The listing builds one solid part. Answer for the finished solid, in the listing's coordinates (mm). A direction names the side the tool comes from. Coordinates: 2 decimals unless noted, no trailing zeros. Order: outer loops, then holes, each group sorted by start corner. A loop starts at its lowest first (then second) coordinate and runs counter-clockwise, first axis right, second up. Notation, with made-up numbers: (-39.75, 85.5) -> (18.25, 85.5) arc R19 ccw to (18.25, 90.5) -> close; hole circle Ø11 at (-30.75, 33). An arc over 180 degrees is marked (long way). Return JSON: item names as keys, results as strings.
```python
from build123d import *

# Parameters (mm, degrees)
SKETCH2_R           = 2.6
SKETCH2_R_2         = 12.75
BOSS_EXTRUDE1_DEPTH = 5
SKETCH3_W           = 115
SKETCH3_H           = 100
BOSS_EXTRUDE2_DEPTH = 5
SKETCH4_W           = 165
SKETCH4_H           = 28.75
BOSS_EXTRUDE3_DEPTH = 5
SKETCH5_W           = 3
SKETCH5_H           = 95
SKETCH5_H_2         = 25
BOSS_EXTRUDE4_DEPTH = 23.75
SKETCH6_R           = 4
CUT_EXTRUDE1_DEPTH  = 5
SKETCH7_R           = 2.55
CUT_EXTRUDE2_DEPTH  = 1
SKETCH8_R           = 2.15
CUT_EXTRUDE3_DEPTH  = 4
SKETCH9_W           = 3
SKETCH9_H           = 28.75
BOSS_EXTRUDE5_DEPTH = 100
CHAMFER1_SIZE       = 70
CHAMFER1_SIZE2      = 28.709092262
FILLET1_R           = 5
FILLET2_R           = 2.5
CUT_EXTRUDE4_DEPTH  = 1.25


with BuildPart() as part:
    # Sketch2 → Boss-Extrude1 (new body)
    with BuildSketch(Plane.XZ.offset(-21.878326304)):
        Polygon((119.866549827, 74.413081659), (14.866549827, 74.413081659), (4.866549827, 74.413081659), (4.866549827, 21.913081659), (14.866549827, 21.913081659), (119.866549827, 21.913081659), align=None)
        Polygon((9.316549827, 34.313081659), (14.316549827, 34.313081659), (26.316549827, 34.313081659), (57.316549827, 34.313081659), (64.316549827, 34.313081659), (64.316549827, 31.013081659), (57.316549753, 31.013081659), (26.316549827, 31.013081659), (14.316549827, 31.013081659), (9.316549827, 31.013081659), align=None, mode=Mode.SUBTRACT)
        with Locations((76.704406531, 39.438081659)):
            Circle(SKETCH2_R, mode=Mode.SUBTRACT)
        with Locations((106.928693123, 39.438081659)):
            Circle(SKETCH2_R, mode=Mode.SUBTRACT)
        Polygon((13.816549827, 59.663081659), (16.816549827, 59.663081659), (59.816549827, 59.663081659), (59.816549827, 36.663081659), (16.816549827, 36.663081659), (13.816549827, 36.663081659), align=None, mode=Mode.SUBTRACT)
        Polygon((57.316549827, 65.313081659), (64.316549827, 65.313081659), (64.316549827, 62.013081659), (57.316549827, 62.013081659), (26.316549827, 62.013081659), (14.316549827, 62.013081659), (9.316549827, 62.013081659), (9.316549827, 65.313081659), (14.316549827, 65.313081659), (26.316549827, 65.313081659), align=None, mode=Mode.SUBTRACT)
        with Locations((91.816549827, 48.163081659)):
            Circle(SKETCH2_R_2, mode=Mode.SUBTRACT)
        with Locations((91.816549827, 65.613081659)):
            Circle(SKETCH2_R, mode=Mode.SUBTRACT)
    extrude(amount=BOSS_EXTRUDE1_DEPTH)

    # Sketch3 → Boss-Extrude2 (add)
    with BuildSketch(Plane(origin=(0, 0, 21.913081659), x_dir=(-1, 0, 0), z_dir=(0, 0, -1))):
        with Locations((-62.366549827, 66.878326304)):
            Rectangle(SKETCH3_W, SKETCH3_H)
    extrude(amount=BOSS_EXTRUDE2_DEPTH)

    # Sketch4 → Boss-Extrude3 (add)
    with BuildSketch(Plane(origin=(0, 116.878326304, 0), x_dir=(1, 0, 0), z_dir=(0, 1, 0))):
        with Locations((62.366549827, -31.288081659)):
            Rectangle(SKETCH4_W, SKETCH4_H)
    extrude(amount=BOSS_EXTRUDE3_DEPTH)

    # Sketch5 → Boss-Extrude4 (add)
    with BuildSketch(Plane.XY.offset(21.913081659)):
        with Locations((65.816549827, 69.378326304)):
            Rectangle(SKETCH5_W, SKETCH5_H)
        with Locations((118.366549827, 104.378326304)):
            Rectangle(SKETCH5_W, SKETCH5_H_2)
        with Locations((118.366549827, 34.378326304)):
            Rectangle(SKETCH5_W, SKETCH5_H_2)
        with Locations((6.366549827, 34.378326304)):
            Rectangle(SKETCH5_W, SKETCH5_H_2)
        with Locations((6.366549827, 104.378326304)):
            Rectangle(SKETCH5_W, SKETCH5_H_2)
    extrude(amount=BOSS_EXTRUDE4_DEPTH)

    # Sketch6 → Cut-Extrude1 (cut)
    with BuildSketch(Plane(origin=(0, 121.878326304, 0), x_dir=(1, 0, 0), z_dir=(0, 1, 0))):
        with Locations((134.866549827, -31.288081659)):
            Circle(SKETCH6_R)
        with Locations((-10.133450173, -31.288081659)):
            Circle(SKETCH6_R)
    extrude(amount=-CUT_EXTRUDE1_DEPTH, mode=Mode.SUBTRACT)

    # Sketch7 → Cut-Extrude2 (cut)
    with BuildSketch(Plane(origin=(0, 0, 16.913081659), x_dir=(-1, 0, 0), z_dir=(0, 0, -1))):
        with Locations((-105.165549827, 90.587326304)):
            Circle(SKETCH7_R)
        with Locations((-105.165549827, 48.423326304)):
            Circle(SKETCH7_R)
        with Locations((-19.821549827, 48.423326304)):
            Circle(SKETCH7_R)
        with Locations((-19.821549827, 90.587326304)):
            Circle(SKETCH7_R)
    extrude(amount=-CUT_EXTRUDE2_DEPTH, mode=Mode.SUBTRACT)

    # Sketch8 → Cut-Extrude3 (cut)
    with BuildSketch(Plane(origin=(0, 0, 17.913081659), x_dir=(-1, 0, 0), z_dir=(0, 0, -1))):
        with Locations((-105.165549827, 90.587326304)):
            Circle(SKETCH8_R)
        with Locations((-19.825549827, 90.587326304)):
            Circle(SKETCH8_R)
        with Locations((-19.825549827, 48.427326304)):
            Circle(SKETCH8_R)
        with Locations((-105.165549827, 48.427326304)):
            Circle(SKETCH8_R)
    extrude(amount=-CUT_EXTRUDE3_DEPTH, mode=Mode.SUBTRACT)

    # Sketch9 → Boss-Extrude5 (add)
    with BuildSketch(Plane(origin=(0, 21.878326304, 0), x_dir=(1, 0, 0), z_dir=(0, 1, 0))):
        with Locations((65.816549827, -60.038081659)):
            Rectangle(SKETCH9_W, SKETCH9_H)
    extrude(amount=BOSS_EXTRUDE5_DEPTH)

    # Chamfer1
    chamfer1_edges = [part.edges().sort_by_distance(p)[0] for p in [
        (65.816549827, 121.878326304, 74.413081659),
    ]]
    chamfer1_side = [part.faces().sort_by_distance(p)[0] for p in [
        (118.309308677, 19.378326304, 74.413081659),
    ]]
    chamfer(chamfer1_edges, length=CHAMFER1_SIZE, length2=CHAMFER1_SIZE2, reference=chamfer1_side[0])

    # Fillet1
    fillet1_edges = [part.edges().sort_by_distance(p)[0] for p in [
        (67.316549827, 116.878326304, 33.788081659),
        (64.316549827, 116.878326304, 33.788081659),
        (118.366549827, 91.878326304, 45.663081659),
        (118.366549827, 91.878326304, 21.913081659),
        (116.866549827, 116.878326304, 33.788081659),
        (118.366549827, 46.878326304, 45.663081659),
        (118.366549827, 46.878326304, 21.913081659),
        (6.366549827, 46.878326304, 45.663081659),
        (6.366549827, 46.878326304, 21.913081659),
        (7.866549827, 116.878326304, 33.788081659),
        (6.366549827, 91.878326304, 45.663081659),
        (6.366549827, 91.878326304, 21.913081659),
        (119.866549827, 19.378326304, 74.413081659),
        (4.866549827, 19.378326304, 74.413081659),
        (119.866549827, 116.878326304, 31.288081659),
        (4.866549827, 116.878326304, 31.288081659),
        (-20.133450173, 119.378326304, 16.913081659),
        (-20.133450173, 119.378326304, 45.663081659),
        (144.866549827, 119.378326304, 45.663081659),
        (144.866549827, 119.378326304, 16.913081659),
    ]]
    fillet(fillet1_edges, radius=FILLET1_R)

    # Fillet2
    fillet2_edges = [part.edges().sort_by_distance(p)[0] for p in [
        (118.366549827, 21.878326304, 45.663081659),
        (6.366549827, 21.878326304, 45.663081659),
        (119.866549827, 16.878326304, 43.163081659),
        (4.866549827, 16.878326304, 43.163081659),
        (62.366549827, 16.878326304, 74.413081659),
        (118.402083733, 16.878326304, 72.948615565),
        (6.331015921, 16.878326304, 72.948615565),
        (62.366549827, 16.878326304, 16.913081659),
    ]]
    fillet(fillet2_edges, radius=FILLET2_R)

    # Sketch10 → Cut-Extrude4 (cut)
    with BuildSketch(Plane(origin=(0, 21.878326304, 0), x_dir=(1, 0, 0), z_dir=(0, 1, 0))):
        Polygon((106.849185334, -35.980469853), (103.894559568, -37.778131521), (103.974067356, -41.235743327), (107.008200912, -42.895693466), (109.962826678, -41.098031798), (109.883318889, -37.640419991), align=None)
        Polygon((73.749780764, -41.235743327), (76.78391432, -42.895693466), (79.738540086, -41.098031798), (79.659032297, -37.640419991), (76.624898742, -35.980469853), (73.670272976, -37.778131521), align=None)
        Polygon((94.850683382, -67.273031798), (94.771175593, -63.815419991), (91.737042038, -62.155469853), (88.782416272, -63.953131521), (88.86192406, -67.410743327), (91.896057616, -69.070693466), align=None)
    extrude(amount=-CUT_EXTRUDE4_DEPTH, mode=Mode.SUBTRACT)


solid = part.part
```
Item 1: Flat-ended cylindrical pins translate along their axes: pin 1 (4 mm diameter, centred on x = 76.7, z = 39.44, fed in from -Y); pin 2 (4.5 mm diameter, centred on x = 19.82, y = 48.42, fed in from +Z); pin 3 (12 mm diameter, centred on x = 41.5, z = 66, fed in from +Y). Find the tip coordinate at first contact, or state that the pin passes through.
Answer list:
{"pin 1": "y = 116.88", "pin 2": "z = 21.91", "pin 3": "y = 21.88"}
Item 2: The part is cut by section D-D on x = 126.5. Determine the outline of the cut face in (y, z), plus the area to 3 significant figures.
Answer list:
{"outline": "(116.88, 16.91) -> (121.88, 16.91) -> (121.88, 45.66) -> (116.88, 45.66) -> close", "area": "144 mm2"}
Item 3: The part is cut by section C-C on y = 108.5. Determine the outline of the cut face in (x, z), plus the area to 3 significant figures.
Answer list:
{"outline": "(4.87, 16.91) -> (119.87, 16.91) -> (119.87, 45.66) -> (116.87, 45.66) -> (116.87, 21.91) -> (67.32, 21.91) -> (67.32, 51.19) -> (64.32, 51.19) -> (64.32, 21.91) -> (7.87, 21.91) -> (7.87, 45.66) -> (4.87, 45.66) -> close", "area": "805 mm2"}
Item 4: Find the intervals of material crossed by probe 1 along X at (y, z) = (44.5, 32.5); probe 2 along Y at (x, z) = (45, 24.5); probe 3 along X at (y, z) = (68, 43), in increasing order.
Answer list:
{"probe 1": "4.87 to 7.87, 64.32 to 67.32, 116.87 to 119.87", "probe 2": "16.88 to 21.88, 116.88 to 121.88", "probe 3": "64.32 to 67.32"}
Item 5: The part is cut by section A-A on x = 40. Determine the outline of the cut face in (y, z).
Answer list:
{"outline": "(16.88, 19.41) arc R2.5 ccw to (19.38, 16.91) -> (121.88, 16.91) -> (121.88, 45.66) -> (116.88, 45.66) -> (116.88, 21.91) -> (21.88, 21.91) -> (21.88, 31.01) -> (16.88, 31.01) -> close; (16.88, 34.31) -> (21.88, 34.31) -> (21.88, 36.66) -> (16.88, 36.66) -> close; (16.88, 59.66) -> (21.88, 59.66) -> (21.88, 62.01) -> (16.88, 62.01) -> close; (16.88, 65.31) -> (21.88, 65.31) -> (21.88, 74.41) -> (19.38, 74.41) arc R2.5 ccw to (16.88, 71.91) -> close"}
Item 6: Which of the six approach directions +Z, -Z, +X, -X, +Y, -Y give full straight-line access (tool end or side, diameter ignored) to faces 1 (the cylindrical face through (6.39, 48.38, 23.34)), 2 (the flat face through (4.867, 62, 20)), 3 (the flat face through (74, 20.628, 38)), 4 (the flat face through (7.867, 102, 34))?
Answer list:
{"face 1": "+Z, -X", "face 2": "+Z, -Z, -X, -Y", "face 3": "none", "face 4": "+Z"}
Item 7: Determine the mould class of faces 5 (the cylindrical face through (3.441, 115.375, 31.087)), 6 (the cylindrical face through (20.29, 46.33, 19.89)), 7 (the flat face through (106, 118, 45.663)) for opening direction Y: pulls with the +Y half, pulls with the -Y half, needs draft (parallel to the pull), parting line crosses it, or undercut.
Answer list:
{"face 5": "pulls with the -Y half", "face 6": "undercut", "face 7": "needs draft"}
Item 8: The part is cut by section B-B on z = 53. Determine the outline of the cut face in (x, y).
Answer list:
{"outline": "(4.87, 19.38) arc R2.5 ccw to (7.37, 16.88) -> (13.82, 16.88) -> (13.82, 21.88) -> (4.87, 21.88) -> close; (59.82, 16.88) -> (80.02, 16.88) -> (80.02, 21.88) -> (67.32, 21.88) -> (67.32, 104.09) -> (64.32, 104.09) -> (64.32, 21.88) -> (59.82, 21.88) -> close; (103.61, 16.88) -> (117.37, 16.88) arc R2.5 ccw to (119.87, 19.38) -> (119.87, 21.88) -> (103.61, 21.88) -> close"}
